Autodesk Inventor part; units mm, degrees
ref_plane "YZ Plane" through (0, 0, 0) normal (1, 0, 0) x (0, 1, 0)
ref_plane "XZ Plane" through (0, 0, 0) normal (0, 1, 0) x (-1, 0, 0)
ref_plane "XY Plane" through (0, 0, 0) normal (0, 0, 1) x (1, 0, 0)
sketch "Sketch1" plane through (0, 0, 0) normal (1, 0, 0) x (0, 1, 0)
  circle A0 centre (0, 0) radius 7.7505
extrude "Extrusion1" add sketch "Sketch1" along normal blind 25
thread "Thread1"
sketch "Sketch2" plane through (0, 0, 0) normal (-1, 0, 0) x (0, 0, 1)
  point P0 (0, 0)
sketch "Sketch3" plane through (0, 0, 0) normal (-1, 0, 0) x (0, 0, 1)
  circle A0 centre (0, 0) radius 10.5233
  line L0 (5.6968, -4.4416) -> (-0.9981, -7.1543)
  line L1 (-0.9981, -7.1543) -> (-6.6949, -2.7128)
  line L2 (-6.6949, -2.7128) -> (-5.6968, 4.4416)
  line L3 (-5.6968, 4.4416) -> (0.9981, 7.1543)
  line L4 (0.9981, 7.1543) -> (6.6949, 2.7128)
  line L5 (6.6949, 2.7128) -> (5.6968, -4.4416)
extrude "Extrusion2" add sketch "Sketch3" along normal blind 15
sketch "Sketch4" plane through (0, 0, 0) normal (-1, 0, 0) x (0, 0, 1)
  point P0 (0, 0)
sketch "Sketch5" plane through (0, 0, 0) normal (-1, 0, 0) x (0, 0, 1)
  point P0 (0, 0)
thread "Thread2"
properties part number "nuts"
The model under review builds one solid part; all positions refer to its coordinate system, in mm. A direction names the side the tool comes from. Round coordinates to 2 decimals unless told otherwise and drop trailing zeros. Order: outer loops, then holes, each group sorted by start corner. A loop starts at its lowest first (then second) coordinate and runs counter-clockwise, first axis right, second up.
Item 1: Draft analysis for pull direction Y (two halves, no side actions). For faces 4 (the flat face through (25, 0, 0)), 5 (the cylindrical face through (12.325, -1.68, 7.566)), 6 (the flat face through (0, 0, 0)), 7 (the flat face through (-7.395, -5.779, 2.396)), state which applies: released by +Y, released by -Y, zero draft, split by the parting line, or undercut.
Working result:
face 4: zero draft
face 5: split by the parting line
face 6: undercut
face 7: undercut
Item 2: Add section D-D, the plane x = 4. State the section outline as (y, z) points.
Working result:
outline: circle Ø15.5 at (0, 0)
Item 3: Add section C-C, the plane y = 0. State the section outline as (x, z) points.
Working result:
outline: (-15, -10.52) - (0, -10.52) - (0, -7.75) - (25, -7.75) - (25, 7.75) - (0, 7.75) - (0, 10.52) - (-15, 10.52) - (-15, 6.32) - (0, 6.32) - (0, -6.32) - (-15, -6.32) - close
Item 4: Machinability: for faces 1 (the flat face through (-7.4, -4.96, -3.81)), 2 (the flat face through (0, -8, -1)), 3 (the cylindrical face through (-7.395, -3.161, 10.037)), which of the approach directions +Z, -Z, +X, -X, +Y, -Y give a long, thin tool a straight path to every point of the face, cutting with its end or side? Answer none if there is none.
Working result:
face 1: -X
face 2: +X
face 3: +X, -X
Item 5: To check wall thickness, follow probe 1 along X at (y, z) = (4.5, 7.75); probe 2 along X at (y, z) = (-1.25, 6); probe 3 along Y at (x, z) = (-2.5, -1.75). State the ranges of each line that lie inside material, in increasing order.
Working result:
probe 1: x = -15 to 0
probe 2: x = 0 to 25
probe 3: y = -10.38 to -6.57, 6.04 to 10.38
Item 6: Add section B-B, the plane z = -3.5. State the section outline as (x, y) points.
Working result:
outline: (-15, -9.92) - (0, -9.92) - (0, -6.92) - (25, -6.92) - (25, 6.92) - (0, 6.92) - (0, 9.92) - (-15, 9.92) - (-15, 5.33) - (0, 5.33) - (0, -5.2) - (-15, -5.2) - close
Item 7: For pin 1 (1.5 mm diameter, centred on x = -6, z = -8.5, fed in from -Y); pin 2 (1.5 mm diameter, centred on x = 16, y = -1.5, fed in from +Z); pin 3 (2 mm diameter, centred on x = 4.5, y = 4.5, fed in from -Z), all flat-tipped, find the tip position at first contact; note any pin that passes through.
Working result:
pin 1: stops at y = -7.12
pin 2: stops at z = 7.71
pin 3: stops at z = -6.92
Item 8: Add section A-A, the plane x = -11. State the section outline as (y, z) points.
Working result:
outline: circle Ø21.05 at (0, 0); hole (-7.15, -1) - (-2.71, -6.69) - (4.44, -5.7) - (7.15, 1) - (2.71, 6.69) - (-4.44, 5.7) - close
